from build123d import *

# Parameters (mm, degrees)
F1_DEPTH = 20


with BuildPart() as f1:
    # F0 (on Front) → F1 (new body)
    with BuildSketch(Plane.XZ):
        with BuildLine():
            ThreePointArc((-30, 29.286612), (-15.810687, -38.829471), (41.925, 0))
            ThreePointArc((41.925, 0), (29.645452, 29.645452), (0, 41.925))
            Line((0, 41.925), (0, 0))
            Line((0, 0), (-30, 0))
            Line((-30, 0), (-30, 29.286612))
        make_face()
        with BuildLine():
            Line((0, 0), (0, 41.925))
            ThreePointArc((0, 41.925), (-16.276738, 38.636426), (-30, 29.286612))
            Line((-30, 29.286612), (-30, 0))
            Line((-30, 0), (0, 0))
        make_face()
        with BuildLine():
            ThreePointArc((-30, 29.286612), (-16.276738, 38.636426), (0, 41.925))
            Line((0, 41.925), (0, 55.575))
            Line((0, 55.575), (-30, 55.575))
            Line((-30, 55.575), (-30, 29.286612))
        make_face()
    extrude(amount=F1_DEPTH)


solid = f1.part
Input: part model. Units: mm. Frame: model coordinates. A direction names the side the tool comes from. Give positions to 0.01 mm unless a question says otherwise; leave off trailing zeros. Write each loop counter-clockwise with the first axis right and the second up, starting at its lowest first coordinate (ties: lowest second). Pieces come first, ordered by that corner, then holes. Notation, with made-up numbers: M -10.75,-2 L 46.25,-2 A18 ccw 46.25,25 Z; hole C 67.5,-32 d6. An arc over 180 degrees is marked long. Use one line per item in the form item = value.
1. Cut plane A-A on y = -3.5. Return loops of the section in (x, z) (3 decimals).
Outcome:
outline = M -30,29.287 A41.925 ccw long 0,41.925 L 0,55.575 L -30,55.575 Z
2. Cut plane B-B on x = -16. Return loops of the section in (y, z) (3 decimals).
Outcome:
outline = M -20,-38.752 L 0,-38.752 L 0,55.575 L -20,55.575 Z
3. First-contact query: P1, Ø5, axis at x = -18, y = -13.5, coming from the -Z side; P2, Ø1.5, axis at y = -6, z = 6, coming from the +X side (3 decimals); P3, Ø6, axis at y = -3.5, z = -7, coming from the -X side. Flat tips, straight axial feed; report the tip coordinate or a pass-through.
Outcome:
P1 = -38.95
P2 = 41.595
P3 = -41.73
4. Ray query, L1, parallel to X at y = -10.5, z = 48; L2, parallel to Z at x = -34, y = -5.5; L3, parallel to X at y = -16.25, z = -7.5. Return the intervals inside material, ascending.
Outcome:
L1 = -30 to 0
L2 = -24.53 to 24.53
L3 = -41.25 to 41.25
5. Reachability of faces 1 (the face through (-1, -20, 8)), 2 (the face through (-30, -10, 43)), 3 (the face through (0, -10, 49)) from +Z, -Z, +X, -X, +Y, -Y: full face, straight path, thin tool, end or side. Return the list, or none.
Outcome:
face_1 = +Z, -Z, +X, -X, -Y
face_2 = +Z, -X, +Y, -Y
face_3 = +Z, +X, +Y, -Y
6. Cut plane C-C on z = 27.5. Return loops of the section in (x, y).
Outcome:
outline = M -31.65,-20 L 31.65,-20 L 31.65,0 L -31.65,0 Z
